Source: CAD feature listing. Evaluate the final solid. Frame: model axes, mm. A direction names the side the tool comes from. Round coordinates to 2 decimals unless told otherwise and drop trailing zeros. Order: outer loops, then holes, each group sorted by start corner. A loop starts at its lowest first (then second) coordinate and runs counter-clockwise, first axis right, second up. Notation, with made-up numbers: (89, -4) -> (121, -4) arc R17 cw to (121, 13) -> close; hole circle Ø3 at (35, 40). An arc over 180 degrees is marked (long way). Answer as CSV lines item,"result".
from build123d import *

# Parameters (mm, degrees)
SKETCH1_W               = 270
SKETCH1_H               = 270
SKETCH1_R               = 7.1
BOSS_EXTRUDE1_DEPTH     = 3
SKETCH2_R               = 1.55
CUT_EXTRUDE1_DEPTH      = 191.942399692
CUT_EXTRUDE2_DEPTH      = 191.942399692
CUT_EXTRUDE2_DEPTH_BACK = 191.942399692
FILLET1_R               = 14.2


with BuildPart() as part:
    # Sketch1 → Boss-Extrude1 (new body)
    with BuildSketch(Plane.XY):
        Rectangle(SKETCH1_W, SKETCH1_H)
        Circle(SKETCH1_R, mode=Mode.SUBTRACT)
        with Locations((-120.8, 120.8)):
            Circle(SKETCH1_R, mode=Mode.SUBTRACT)
        with Locations(Location((-120.8, -120.8, 0), (0, 0, 180))):
            Circle(SKETCH1_R, mode=Mode.SUBTRACT)
        with Locations((120.8, -120.8)):
            Circle(SKETCH1_R, mode=Mode.SUBTRACT)
        with Locations(Location((120.8, 120.8, 0), (0, 0, 180))):
            Circle(SKETCH1_R, mode=Mode.SUBTRACT)
        with Locations((-96.051262658, 96.051262658)):
            Circle(SKETCH1_R, mode=Mode.SUBTRACT)
        with Locations((-71.302525317, 71.302525317)):
            Circle(SKETCH1_R, mode=Mode.SUBTRACT)
        with Locations((-46.553787975, 46.553787975)):
            Circle(SKETCH1_R, mode=Mode.SUBTRACT)
        with Locations(Location((46.553787975, 46.553787975, 0), (0, 0, 180))):
            Circle(SKETCH1_R, mode=Mode.SUBTRACT)
        with Locations(Location((71.302525317, 71.302525317, 0), (0, 0, 180))):
            Circle(SKETCH1_R, mode=Mode.SUBTRACT)
        with Locations(Location((96.051262658, 96.051262658, 0), (0, 0, 180))):
            Circle(SKETCH1_R, mode=Mode.SUBTRACT)
        with Locations((96.051262658, -96.051262658)):
            Circle(SKETCH1_R, mode=Mode.SUBTRACT)
        with Locations((71.302525317, -71.302525317)):
            Circle(SKETCH1_R, mode=Mode.SUBTRACT)
        with Locations((46.553787975, -46.553787975)):
            Circle(SKETCH1_R, mode=Mode.SUBTRACT)
        with Locations(Location((-46.553787975, -46.553787975, 0), (0, 0, 180))):
            Circle(SKETCH1_R, mode=Mode.SUBTRACT)
        with Locations(Location((-71.302525317, -71.302525317, 0), (0, 0, 180))):
            Circle(SKETCH1_R, mode=Mode.SUBTRACT)
        with Locations(Location((-96.051262658, -96.051262658, 0), (0, 0, 180))):
            Circle(SKETCH1_R, mode=Mode.SUBTRACT)
    extrude(amount=BOSS_EXTRUDE1_DEPTH)

    # Sketch2 → Cut-Extrude1 (cut, symmetric)
    with BuildSketch(Plane.XY):
        with Locations((-28, 13)):
            Circle(SKETCH2_R)
        with Locations(Location((-28, -13, 0), (0, 0, 180))):
            Circle(SKETCH2_R)
        with Locations((-28, 26)):
            Circle(SKETCH2_R)
        with Locations(Location((-28, -26, 0), (0, 0, 180))):
            Circle(SKETCH2_R)
        with Locations((28, -26)):
            Circle(SKETCH2_R)
        with Locations(Location((28, 26, 0), (0, 0, 180))):
            Circle(SKETCH2_R)
    cut_extrude1 = extrude(amount=CUT_EXTRUDE1_DEPTH, both=True, mode=Mode.SUBTRACT)

    # Mirror1: Cut-Extrude1 across plane
    add(cut_extrude1.mirror(Plane(origin=(0, 0, 0), x_dir=(0, 0, 1), z_dir=(1, 0, 0))), mode=Mode.SUBTRACT)

    # Sketch4 → Cut-Extrude2 (cut, two sides: drawn at the far end of the back side and taken through both)
    with BuildSketch(Plane.XY.offset(-CUT_EXTRUDE2_DEPTH_BACK)):
        Polygon((-135, 115), (-93.526641242, 71.641488571), (-93.526641242, -71.641488571), (-135, -115), align=None)
        Polygon((115, 135), (-115, 135), (-71.641488571, 93.526641242), (71.641488571, 93.526641242), align=None)
        Polygon((135, -115), (135, 115), (93.526641242, 71.641488571), (93.526641242, -71.641488571), align=None)
        Polygon((115, -135), (71.641488571, -93.526641242), (-71.641488571, -93.526641242), (-115, -135), align=None)
        Polygon((-78, 55.409090909), (-78, -55.409090909), (-25, 0), align=None)
        Polygon((55.409090909, 78), (-55.409090909, 78), (0, 25), align=None)
        Polygon((78, -55.409090909), (78, 55.409090909), (25, 0), align=None)
        Polygon((-55.409090909, -78), (55.409090909, -78), (0, -25), align=None)
    extrude(amount=CUT_EXTRUDE2_DEPTH + CUT_EXTRUDE2_DEPTH_BACK, mode=Mode.SUBTRACT)

    # Fillet1
    fillet1_edges = [part.edges().sort_by_distance(p)[0] for p in [
        (93.526641242, 71.641488571, 1.5),
        (135, -115, 1.5),
        (135, 115, 1.5),
        (93.526641242, -71.641488571, 1.5),
        (0, 25, 1.5),
        (55.409090909, 78, 1.5),
        (-55.409090909, 78, 1.5),
        (-71.641488571, 93.526641242, 1.5),
        (115, 135, 1.5),
        (-115, 135, 1.5),
        (71.641488571, 93.526641242, 1.5),
        (-78, -55.409090909, 1.5),
        (-25, 0, 1.5),
        (-78, 55.409090909, 1.5),
        (0, -25, 1.5),
        (-55.409090909, -78, 1.5),
        (55.409090909, -78, 1.5),
        (-115, -135, 1.5),
        (71.641488571, -93.526641242, 1.5),
        (115, -135, 1.5),
        (-71.641488571, -93.526641242, 1.5),
        (25, 0, 1.5),
        (78, -55.409090909, 1.5),
        (78, 55.409090909, 1.5),
        (-135, 115, 1.5),
        (-93.526641242, -71.641488571, 1.5),
        (-135, -115, 1.5),
        (-93.526641242, 71.641488571, 1.5),
        (135, -135, 1.5),
        (-135, -135, 1.5),
        (-135, 135, 1.5),
        (135, 135, 1.5),
    ]]
    fillet(fillet1_edges, radius=FILLET1_R)


solid = part.part
1. Pin query (flat end, axial travel): pin 1 (3 mm diameter, centred on x = -28, y = -13, fed in from -Z); pin 2 (1.5 mm diameter, centred on x = -95, z = 2.5, fed in from +Y); pin 3 (1.5 mm diameter, centred on y = 4, z = 1, fed in from +X); pin 4 (1.5 mm diameter, centred on x = 34, z = 1.5, fed in from -Y). Return the tip coordinate at first contact, or that it passes through.
Results below:
pin 1,"through"
pin 2,"y = 116.59"
pin 3,"x = 93.53"
pin 4,"y = -93.53"
2. Line query: L1, parallel to Y at x = 99, z = 1.3; L2, parallel to Y at x = 97, z = 1.5; L3, parallel to X at y = -8.5, z = 2.4. Output: solid intervals per line, ascending. Write a range as [from, to].
Results below:
L1,"[-119.7, -102.51], [-89.59, -77.36], [77.36, 89.59], [102.51, 119.7]"
L2,"[-117.78, -103.09], [-89.01, -75.25], [75.25, 89.01], [103.09, 117.78]"
L3,"[-93.53, -78], [-33.28, 33.28], [78, 93.53]"
3. Section query C-C on y = -61. Return loops of the section in (x, z).
Results below:
outline,"(-93.53, 0) -> (-33.94, 0) -> (-33.94, 3) -> (-93.53, 3) -> close; (33.94, 0) -> (93.53, 0) -> (93.53, 3) -> (33.94, 3) -> close"
4. Section query A-A on y = 0. Return loops of the section in (x, z), and give its area (3 significant figures).
Results below:
outline,"(-93.53, 0) -> (-78, 0) -> (-78, 3) -> (-93.53, 3) -> close; (-30.45, 0) -> (-7.1, 0) -> (-7.1, 3) -> (-30.45, 3) -> close; (7.1, 0) -> (30.45, 0) -> (30.45, 3) -> (7.1, 3) -> close; (78, 0) -> (93.53, 0) -> (93.53, 3) -> (78, 3) -> close"
area,"233 mm2"
5. Mould query, pull axis Y, two halves, no side actions, for faces 4 (the cylindrical face through (130.73, 130.95, 1.52)), 5 (the flat face through (-93.075, -114.028, 1.479)), 6 (the cylindrical face through (-121.72, 127.84, 1.48)). Classes: released by +Y, released by -Y, zero draft, split by the parting line, or undercut.
Results below:
face 4,"released by +Y"
face 5,"released by -Y"
face 6,"undercut"
6. Section query D-D on z = 1.4. Give the number of separate pieces and of enclosed holes in the cut face, and give its area (3 significant figures).
Results below:
separate pieces,"1"
enclosed holes,"29"
area,"29,500 mm2"
7. Reachability of faces 1 (the flat face through (28, 2, 0)), 2 (the flat face through (-114.5, 93.57, 1.48)), 3 (the flat face through (43.829, -19.685, 1.479)) from +Z, -Z, +X, -X, +Y, -Y: full face, straight path, thin tool, end or side. Return the list, or none.
Results below:
face 1,"-Z, +X, -X, +Y, -Y"
face 2,"+Z, -Z, -X"
face 3,"+Z, -Z"
8. Section query B-B on x = -58. Return loops of the section in (y, z), and give its area (3 significant figures).
Results below:
outline,"(-93.53, 0) -> (-32.98, 0) -> (-32.98, 3) -> (-93.53, 3) -> close; (32.98, 0) -> (93.53, 0) -> (93.53, 3) -> (32.98, 3) -> close"
area,"363 mm2"
